Geometry check sheet. Reference: the model listing, model coordinates, mm. Face numbers are marked on the shaded views. A direction names the side the tool comes from. Give positions to 0.01 mm unless a question says otherwise; leave off trailing zeros. Order: outer loops, then holes, each group sorted by start corner. A loop starts at its lowest first (then second) coordinate and runs counter-clockwise, first axis right, second up. Notation, with made-up numbers: M 65,75 L 115,75 A24 cw 115,104 Z; hole C -14,49 d9. An arc over 180 degrees is marked long. Put each result on its own line as item: value. Start each with the question number.
Q1. Access from +Z, -Z, +X, -X, +Y, -Y to the whole of each face (thin tool, end or side, straight path). Record for the marked faces 4, 5 and 6.
Q2. Section check A-A on y = -131.5. Record the cut outline in (x, z).
Q3. Material ranges on L1, parallel to Z at x = 117, y = -115; L2, parallel to X at y = -80, z = 462.5; L3, parallel to Y at x = 255.5, z = 617, recorded low to high.
Q4. Section check B-B on x = 120.5. Record the cut outline in (y, z), then the cut area to 3 significant figures.
Q5. Go/stop test with flat-tipped pins: pin 1 (10 mm diameter, centred on x = 234, z = 692.5, fed in from +Y); pin 2 (5 mm diameter, centred on x = 158, z = 471.5, fed in from -Y); pin 3 (1 mm diameter, centred on y = -116.5, z = 206.5, fed in from +X). Record where each tip stops, or that it passes through.
Q6. Section check C-C on z = 567.5. Record the cut outline in (x, y).
Q7. Section check D-D on y = -73.5. Record the cut outline in (x, z).
Q8. Mould release check, pull along X, two halves, no side actions. Record for the marked faces 1, 2 and 3: +X half, -X half, draft (parallel to the pull), parting line (faces both ways), or undercut.
```python
from build123d import *

# Parameters (mm, degrees)
F0_W     = 609.6
F0_H     = 914.4
F1_DEPTH = 25.4
F2_W     = 177.8
F2_H     = 914.4
F3_DEPTH = 127
F4_W     = 152.4
F4_H     = 889
F5_DEPTH = 101.6
F6_W     = 152.4
F6_H     = 12.7
F7_DEPTH = 101.6
F9_DEPTH = 12.7


with BuildPart() as f1:
    # F0 (on Front) → F1 (new body)
    with BuildSketch(Plane.XZ):
        with Locations((304.8, 457.2)):
            Rectangle(F0_W, F0_H)
    extrude(amount=F1_DEPTH)

    # F2 (on face) → F3 (join)
    with BuildSketch(Plane.XZ.offset(25.4)):
        with Locations((88.9, 457.2)):
            Rectangle(F2_W, F2_H)
    extrude(amount=F3_DEPTH)

    # F4 (on face) → F5 (cut)
    with BuildSketch(Plane.XZ.offset(152.4)):
        with Locations((88.9, 457.2)):
            Rectangle(F4_W, F4_H)
    extrude(amount=-F5_DEPTH, mode=Mode.SUBTRACT)

    # F6 (on face) → F7 (join)
    with BuildSketch(Plane.XZ.offset(50.8)):
        with Locations((88.9, 666.75)):
            Rectangle(F6_W, F6_H)
        with Locations((88.9, 527.05)):
            Rectangle(F6_W, F6_H)
        with Locations((88.9, 387.35)):
            Rectangle(F6_W, F6_H)
        with Locations((88.9, 260.35)):
            Rectangle(F6_W, F6_H)
    extrude(amount=F7_DEPTH)

    # F8 (on Top) → F9 (join)
    with BuildSketch(Plane.XY):
        Polygon((177.8, -25.4), (177.8, -152.4), (609.6, -25.4), align=None)
    extrude(amount=F9_DEPTH)


solid = f1.part
```
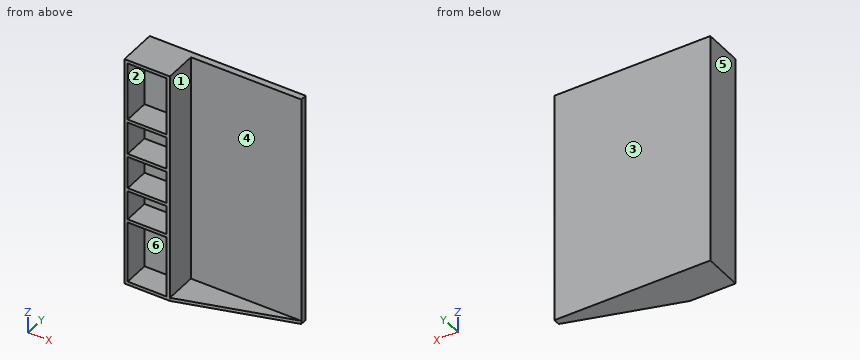
Results found:
1. face 4: +Z, +X, -Y
1. face 5: +Z, -Z, -X, +Y, -Y
1. face 6: -Y
2. outline: M 0,0 L 248.86,0 L 248.86,12.7 L 177.8,12.7 L 177.8,914.4 L 0,914.4 Z; hole M 12.7,12.7 L 165.1,12.7 L 165.1,254 L 12.7,254 Z; hole M 12.7,266.7 L 165.1,266.7 L 165.1,381 L 12.7,381 Z; hole M 12.7,393.7 L 165.1,393.7 L 165.1,520.7 L 12.7,520.7 Z; hole M 12.7,533.4 L 165.1,533.4 L 165.1,660.4 L 12.7,660.4 Z; hole M 12.7,673.1 L 165.1,673.1 L 165.1,901.7 L 12.7,901.7 Z
3. L1: z = 0 to 12.7, 254 to 266.7, 381 to 393.7, 520.7 to 533.4, 660.4 to 673.1, 901.7 to 914.4
3. L2: x = 0 to 12.7, 165.1 to 177.8
3. L3: y = -25.4 to 0
4. outline: M -152.4,0 L 0,0 L 0,914.4 L -152.4,914.4 L -152.4,901.7 L -50.8,901.7 L -50.8,673.1 L -152.4,673.1 L -152.4,660.4 L -50.8,660.4 L -50.8,533.4 L -152.4,533.4 L -152.4,520.7 L -50.8,520.7 L -50.8,393.7 L -152.4,393.7 L -152.4,381 L -50.8,381 L -50.8,266.7 L -152.4,266.7 L -152.4,254 L -50.8,254 L -50.8,12.7 L -152.4,12.7 Z
4. area: 54,200 mm^2
5. pin 1: stops at y = 0
5. pin 2: stops at y = -50.8
5. pin 3: stops at x = 177.8
6. outline: M 0,-152.4 L 12.7,-152.4 L 12.7,-50.8 L 165.1,-50.8 L 165.1,-152.4 L 177.8,-152.4 L 177.8,-25.4 L 609.6,-25.4 L 609.6,0 L 0,0 Z
7. outline: M 0,0 L 446.06,0 L 446.06,12.7 L 177.8,12.7 L 177.8,914.4 L 0,914.4 Z; hole M 12.7,12.7 L 165.1,12.7 L 165.1,254 L 12.7,254 Z; hole M 12.7,266.7 L 165.1,266.7 L 165.1,381 L 12.7,381 Z; hole M 12.7,393.7 L 165.1,393.7 L 165.1,520.7 L 12.7,520.7 Z; hole M 12.7,533.4 L 165.1,533.4 L 165.1,660.4 L 12.7,660.4 Z; hole M 12.7,673.1 L 165.1,673.1 L 165.1,901.7 L 12.7,901.7 Z
8. face 1: +X half
8. face 2: undercut
8. face 3: draft
